```python
from build123d import *

# Parameters (mm, degrees)
F0_R     = 2
F1_DEPTH = 5


# Not quite as in the source:
# - ends of sketch curves that miss each other by under 0.0002 mm in the source are joined


with BuildPart() as f1:
    # F0 (on Top) → F1 (new body)
    with BuildSketch(Plane.XY):
        with BuildLine():
            ThreePointArc((-86.9239089763, -96.6023878966), (-99.0303580955, -105.1836331247), (-89.144034, -116.25))
            Line((-89.144034, -116.25), (86.235345, -116.25))
            ThreePointArc((86.235345, -116.25), (96.1216690408, -105.1836326404), (84.0152190261, -96.6023881141))
            Line((84.0152190261, -96.6023881141), (78.54514, -97.854584))
            Line((78.54514, -97.854584), (71.133383, -98.793694))
            Line((71.133383, -98.793694), (64.939287, -99.095039))
            Line((64.939287, -99.095039), (58.739872, -98.995936))
            Line((58.739872, -98.995936), (52.07042, -98.463421))
            Line((52.07042, -98.463421), (45.452353, -97.494386))
            Line((45.452353, -97.494386), (37.288225, -95.647643))
            Line((37.288225, -95.647643), (29.552302, -92.435031))
            Line((29.552302, -92.435031), (23.41918, -88.534685))
            Line((23.41918, -88.534685), (17.86875, -83.821678))
            Line((17.86875, -83.821678), (13.197325, -78.879824))
            Line((13.197325, -78.879824), (9.083287, -73.477642))
            Line((9.083287, -73.477642), (7.586324, -70.18701))
            ThreePointArc((7.586324, -70.18701), (-1.454345, -64.321401), (-10.4950136906, -70.1870101381))
            Line((-10.4950136906, -70.1870101381), (-11.991976, -73.477642))
            Line((-11.991976, -73.477642), (-16.106015, -78.879824))
            Line((-16.106015, -78.879824), (-20.77744, -83.821678))
            Line((-20.77744, -83.821678), (-26.32787, -88.534685))
            Line((-26.32787, -88.534685), (-32.460992, -92.435031))
            Line((-32.460992, -92.435031), (-40.196915, -95.647643))
            Line((-40.196915, -95.647643), (-48.361042, -97.494386))
            Line((-48.361042, -97.494386), (-54.979109, -98.463421))
            Line((-54.979109, -98.463421), (-61.648561, -98.995936))
            Line((-61.648561, -98.995936), (-67.847977, -99.095039))
            Line((-67.847977, -99.095039), (-74.042073, -98.793694))
            Line((-74.042073, -98.793694), (-81.45383, -97.854584))
            Line((-81.45383, -97.854584), (-86.9239089763, -96.6023878966))
        make_face()
        with Locations((-88.954345, -106.25)):
            Circle(F0_R, mode=Mode.SUBTRACT)
        with Locations((86.045655, -106.25)):
            Circle(F0_R, mode=Mode.SUBTRACT)
    extrude(amount=F1_DEPTH)


solid = f1.part
```
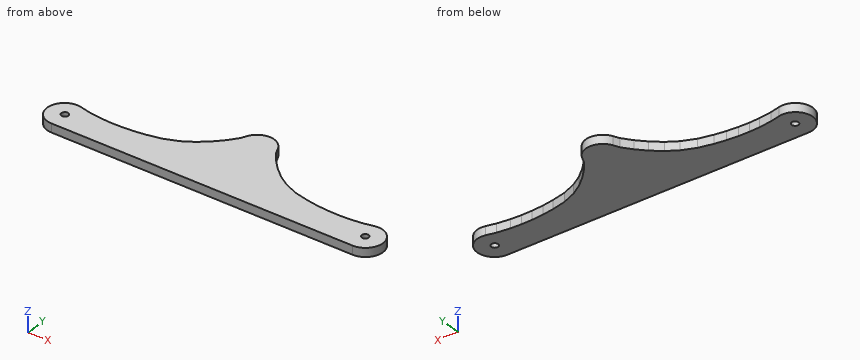
Part model, mm, in its own coordinate system. Coordinates: 2 decimals unless noted, no trailing zeros. Write each loop counter-clockwise with the first axis right and the second up, starting at its lowest first coordinate (ties: lowest second). Pieces come first, ordered by that corner, then holes.
Item 1: Pin check, flat tips, straight feed: pin 1 (4.5 mm diameter, centred on x = 86.05, y = -106.25, fed in from +Z); pin 2 (1 mm diameter, centred on y = -99.5, z = 2.5, fed in from +X); pin 3 (3.5 mm diameter, centred on x = -88.95, y = -106.25, fed in from +Z); pin 4 (3 mm diameter, centred on y = -82.5, z = 0.5, fed in from +X). Stop position of each tip, or through.
Item 2: Slice it at D-D (y = -76.5). Write the cut outline in (x, z).
Item 3: Slice it at B-B (y = -106.25). Write the cut outline in (x, z).
Item 4: Probe line 1 (X direction, y = -105, z = 2.5); line 2 (Y direction, x = 41.5, z = 1.05); line 3 (Y direction, x = 4.5, z = 3.9). List the from-to ranges inside material, lowest first.
Item 5: Slice it at A-A (z = 3.1). Count the separate pieces of the cut face and the enclosed holes in it, and give its area (3 significant figures).
Item 6: Slice it at C-C (x = -44.5). Write the cut outline in (y, z), and give its area (3 significant figures).
Results found:
1. pin 1: stops at z = 5
1. pin 2: stops at x = 93.94
1. pin 3: passes through
1. pin 4: stops at x = 18.08
2. outline: (-14.29, 0) - (11.38, 0) - (11.38, 5) - (-14.29, 5) - close
3. outline: (-99.09, 0) - (-90.95, 0) - (-90.95, 5) - (-99.09, 5) - close; (-86.95, 0) - (84.05, 0) - (84.05, 5) - (-86.95, 5) - close; (88.05, 0) - (96.18, 0) - (96.18, 5) - (88.05, 5) - close
4. line 1: x = -99.01 to -90.52, -87.39 to 84.48, 87.61 to 96.1
4. line 2: y = -116.25 to -96.6
4. line 3: y = -116.25 to -66.31
5. separate pieces: 1
5. enclosed holes: 2
5. area: 4,760 mm2
6. outline: (-116.25, 0) - (-96.62, 0) - (-96.62, 5) - (-116.25, 5) - close
6. area: 98.1 mm2
